Source: CAD feature listing. Evaluate the final solid. Frame: model axes, mm. Round coordinates to 2 decimals unless told otherwise and drop trailing zeros. Loops run counter-clockwise (first coordinate to the right, second up) from the corner with the lowest first, then second, coordinate; pieces in that order, holes last. Notation, with made-up numbers: (18, 3) -> (47, 3) arc R27 cw to (47, 32) -> close; hole circle Ø6 at (77.5, 45.25). An arc over 180 degrees is marked (long way). Return JSON: item names as keys, results as strings. Group by question number.
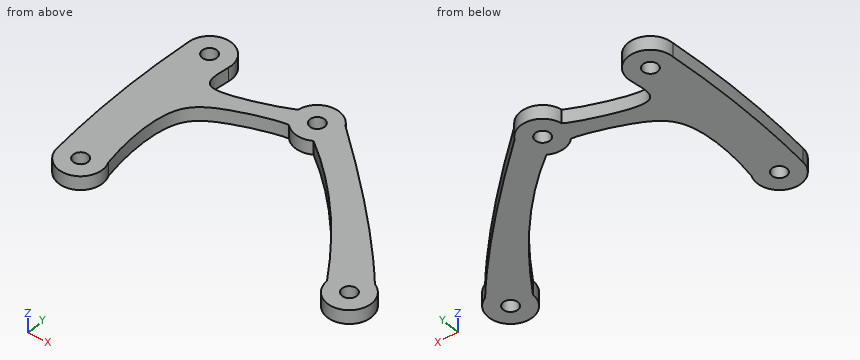
Autodesk Inventor part; units mm, degrees
ref_plane "YZ Plane" through (0, 0, 0) normal (1, 0, 0) x (0, 1, 0)
ref_plane "XZ Plane" through (0, 0, 0) normal (0, 1, 0) x (-1, 0, 0)
ref_plane "XY Plane" through (0, 0, 0) normal (0, 0, 1) x (1, 0, 0)
sketch "Sketch1" plane through (0, 0, 0) normal (0, 0, 1) x (1, 0, 0)
  line L0 (-110, 70) -> (110, 70) construction
  line L1 (110, 70) -> (110, -70) construction
  line L2 (110, -70) -> (-110, -70) construction
  line L3 (-110, -70) -> (-110, 70) construction
  circle A0 centre (-90, 55) radius 5
  circle A1 centre (-90, -55) radius 5
  circle A2 centre (90, -55) radius 5
  circle A3 centre (-10, 45) radius 5
  line L4 (-67, 0) -> (-42, 0) construction
  line L5 (-42, 0) -> (-42, -30) construction
  line L6 (-42, -30) -> (-67, -30) construction
  line L7 (-67, -30) -> (-67, 0) construction
  circle A4 centre (-54.5, -11) radius 10 construction
  circle A5 centre (-63.5044, -24.4163) radius 3 construction
  circle A6 centre (-57.3559, -26.4695) radius 3 construction
  circle A7 centre (-51.263, -24.6531) radius 3 construction
  circle A8 centre (-45.3418, -26.5938) radius 3 construction
  arc A9 (-75.2459, 52.2951) -> (-105, 55) centre (-90, 55) ccw
  arc A10 (-104.9399, -56.3418) -> (-76.4307, -48.6067) centre (-90, -55) ccw
  arc A11 (75, -55) -> (96.4821, -41.4729) centre (90, -55) ccw
  line L8 (-105, 55) -> (-110, 0) construction
  line L9 (-110, 0) -> (-104.9399, -56.3418) construction
  spline S0 degree 2 poles (-105, 55) (-110, 0) (-104.9399, -56.3418) knots 1 1 1 2 2 2
  line L10 (-75.2459, 52.2951) -> (-77.8614, 38.0288) construction
  line L11 (-77.8614, 38.0288) -> (-75, 30.9694) construction
  line L12 (-75, 30.9694) -> (-62.6528, 32.0783) construction
  line L13 (-62.6528, 32.0783) -> (-28.1231, 45) construction
  line L14 (-28.1231, 45) -> (-24.7541, 47.7049) construction
  spline S1 degree 4 poles (-75.2459, 52.2951) (-77.8614, 38.0288) (-75, 30.9694) (-62.6528, 32.0783) (-28.1231, 45) (-24.7541, 47.7049) knots 1 1 1 1 1 2 3 3 3 3 3
  line L15 (-76.4307, -48.6067) -> (-79.8699, -29.5938) construction
  line L16 (-79.8699, -29.5938) -> (-79.8699, 0) construction
  line L17 (-79.8699, 0) -> (-73.4228, 13.4087) construction
  line L18 (-73.4228, 13.4087) -> (-61.869, 23.3517) construction
  line L19 (-61.869, 23.3517) -> (-26.4386, 34.4991) construction
  line L20 (-26.4386, 34.4991) -> (-20.7113, 34.4991) construction
  spline S2 degree 4 poles (-76.4307, -48.6067) (-79.8699, -29.5938) (-79.8699, 0) (-73.4228, 13.4087) (-61.869, 23.3517) (-26.4386, 34.4991) (-20.7113, 34.4991) knots 1 1 1 1 1 2 3 4 4 4 4 4
  line L21 (-2.3823, 32.0783) -> (40.3668, 0) construction
  line L22 (40.3668, 0) -> (75, -55) construction
  spline S3 degree 2 poles (-2.3823, 32.0783) (40.3668, 0) (75, -55) knots 1 1 1 2 2 2
  line L23 (3.1066, 52.2951) -> (62.3, 0) construction
  line L24 (62.3, 0) -> (96.4821, -41.4729) construction
  spline S4 degree 2 poles (3.1066, 52.2951) (62.3, 0) (96.4821, -41.4729) knots 1 1 1 2 2 2
  arc A12 (-20.7113, 34.4991) -> (-2.3823, 32.0783) centre (-10, 45) ccw
  arc A13 (3.1066, 52.2951) -> (-24.7541, 47.7049) centre (-10, 45) ccw
  point P0 (0, 0)
  dimension "d1" = 70
  dimension "d2" = 70
  dimension "d3" = 110
  dimension "d4" = 110
  dimension "d5" = 10
  dimension "d6" = 10
  dimension "d7" = 10
  dimension "d8" = 10
  dimension "d9" = 55
  dimension "d10" = 55
  dimension "d11" = 55
  dimension "d12" = 180
  dimension "d13" = 90
  dimension "d14" = 90
  dimension "d15" = 10
  dimension "d16" = 45
  dimension "d17" = 42
  dimension "d18" = 30
  dimension "d19" = 0
  dimension "d20" = 25
  dimension "d21" = 20
  dimension "d22" = 6
  dimension "d23" = 6
  dimension "d24" = 6
  dimension "d25" = 11
  dimension "d26" = 12.5
  dimension "d27" = 6
  dimension "d42" = 30
  dimension "d43" = 30
extrude "Extrusion3" add sketch "Sketch1" along normal blind 9.4
equation "\"d26\" = 0.5 * d20"
properties part number "Bracket Concept MK4"
(1) Ray query, line 1 (Y direction, x = -90, z = 6.5); line 2 (Y direction, x = -9.5, z = 5.5); line 3 (X direction, y = -12, z = 8.75). Return the intervals inside material, ascending.
(2) Cut plane C-C (z = 5.75). Count the separate pieces of the cut face and the enclosed holes in it, and give its area (3 significant figures).
(3) Cut plane B-B (x = -10). Return loops of the section in (y, z), and give its area (3 significant figures).
(4) Pin query (flat end, axial travel): pin 1 (8 mm diameter, centred on x = -90, y = -55, fed in from +Z); pin 2 (8 mm diameter, centred on x = -41, y = 37.5, fed in from -Z); pin 3 (5 mm diameter, centred on x = -20.5, z = 6, fed in from +Y); pin 4 (5 mm diameter, centred on y = 22, z = 2.5, fed in from +X). Return the tip coordinate at first contact, or that it passes through.
(5) Cut plane A-A (x = -90). Return loops of the section in (y, z), and give its area (3 significant figures).
Answers follow:
{
 "1": {"line 1": "-70 to -60, -50 to 50, 60 to 70", "line 2": "30.01 to 40.03, 49.97 to 59.99", "line 3": "-107.37 to -79, 43.77 to 70.33"},
 "2": {"separate pieces": "1", "enclosed holes": "4", "area": "8,080 mm^2"},
 "3": {"outline": "(30, 0) -> (40, 0) -> (40, 9.4) -> (30, 9.4) -> close; (50, 0) -> (60, 0) -> (60, 9.4) -> (50, 9.4) -> close", "area": "188 mm^2"},
 "4": {"pin 1": "through", "pin 2": "z = 0", "pin 3": "y = 57.69", "pin 4": "x = 38.88"},
 "5": {"outline": "(-70, 0) -> (-60, 0) -> (-60, 9.4) -> (-70, 9.4) -> close; (-50, 0) -> (50, 0) -> (50, 9.4) -> (-50, 9.4) -> close; (60, 0) -> (70, 0) -> (70, 9.4) -> (60, 9.4) -> close", "area": "1,130 mm^2"}
}
